```python
from build123d import *

# Parameters (mm, degrees)
F0_R     = 10.25
F0_R_2   = 7.5
F1_DEPTH = 40
F2_R     = 10.25
F2_R_2   = 7.5
F2_R_3   = 2
F3_DEPTH = 5
F4_R     = 2


with BuildPart() as f1:
    # F0 (on Front) → F1 (new body)
    with BuildSketch(Plane.XZ):
        Circle(F0_R)
        Circle(F0_R_2, mode=Mode.SUBTRACT)
    extrude(amount=-F1_DEPTH)

    # F2 (on face) → F3 (join)
    with BuildSketch(Plane(origin=(0, 40, 0), x_dir=(-1, 0, 0), z_dir=(0, 1, 0))):
        Circle(F2_R)
        Circle(F2_R_2, mode=Mode.SUBTRACT)
        Circle(F2_R_2)
        Circle(F2_R_3, mode=Mode.SUBTRACT)
    extrude(amount=-F3_DEPTH)

    # F4
    f4_edges = [f1.edges().sort_by_distance(p)[0] for p in [
        (2, 35, 0),
    ]]
    fillet(f4_edges, radius=F4_R)


solid = f1.part
```
The listing builds one solid part. Answer for the finished solid, in the listing's coordinates (mm). Round coordinates to 2 decimals unless told otherwise and drop trailing zeros. Loops run counter-clockwise (first coordinate to the right, second up) from the corner with the lowest first, then second, coordinate; pieces in that order, holes last.
1) A cutting plane is placed at D-D on z = -6. Determine the outline of the cut face in (x, y).
Outcome:
outline: (-8.31, 0) - (-4.5, 0) - (-4.5, 35) - (4.5, 35) - (4.5, 0) - (8.31, 0) - (8.31, 40) - (-8.31, 40) - close
2) For a pull along X with two mould halves and no side action, classify faces 1 (the face through (-2.222, 19.72, -10.006)), 2 (the face through (-7.493, 17.255, 0.33)), 3 (the face through (1, 0, -8)), 4 (the face through (-3, 35, -3)) as released by +X, released by -X, zero draft, split by the parting line, or undercut.
Outcome:
face 1: split by the parting line
face 2: undercut
face 3: zero draft
face 4: undercut
3) A cutting plane is placed at B-B on z = 0. Determine the outline of the cut face in (x, y), plus the area to 3 significant figures.
Outcome:
outline: (-10.25, 0) - (-7.5, 0) - (-7.5, 35) - (-4, 35) arc R2 ccw to (-2, 37) - (-2, 40) - (-10.25, 40) - close; (2, 37) arc R2 ccw to (4, 35) - (7.5, 35) - (7.5, 0) - (10.25, 0) - (10.25, 40) - (2, 40) - close
area: 273 mm2
4) A cutting plane is placed at C-C on y = 33. Determine the outline of the cut face in (x, z).
Outcome:
outline: circle Ø20.5 at (0, 0); hole circle Ø15 at (0, 0)
5) Given P1, Ø2, axis at y = 15.5, z = -3.5, coming from the +X side; P2, Ø4, axis at y = 35.5, z = -7, coming from the -X side; P3, Ø1.5, axis at x = 3, y = 30.5, coming from the -Z side, each flat-ended and moving along its own axis, determine where each tip first touches the part or whether it passes through.
Outcome:
P1: stops at x = 9.94
P2: stops at x = -8.95
P3: stops at z = -10
6) A cutting plane is placed at A-A on x = 0. Determine the outline of the cut face in (y, z).
Outcome:
outline: (0, -10.25) - (40, -10.25) - (40, -2) - (37, -2) arc R2 ccw to (35, -4) - (35, -7.5) - (0, -7.5) - close; (0, 7.5) - (35, 7.5) - (35, 4) arc R2 ccw to (37, 2) - (40, 2) - (40, 10.25) - (0, 10.25) - close
7) Consider line 1 (Z direction, x = 0, y = 13); line 2 (X direction, y = 30, z = -4.5); line 3 (X direction, y = 12, z = 4). Determine where each line is inside the solid, lowest interval first.
Outcome:
line 1: z = -10.25 to -7.5, 7.5 to 10.25
line 2: x = -9.21 to -6, 6 to 9.21
line 3: x = -9.44 to -6.34, 6.34 to 9.44
